Could you check a few things on this model? Use its own coordinates, in mm. Face numbers are marked on the shaded views. A direction names the side the tool comes from. Give positions to 0.01 mm unless a question says otherwise; leave off trailing zeros. Order: outer loops, then holes, each group sorted by start corner. A loop starts at its lowest first (then second) coordinate and runs counter-clockwise, first axis right, second up.
from build123d import *

# Parameters (mm, degrees)
F0_R     = 25
F1_DEPTH = 88
F3_DEPTH = 50
F5_DEPTH = 16
F7_R     = 6
F8_DEPTH = 9


with BuildPart() as f1:
    # F0 (on Top) → F1 (new body)
    with BuildSketch(Plane.XY):
        with BuildLine():
            Line((0, 75), (0, 0))
            Line((0, 0), (50, 0))
            ThreePointArc((50, 0), (87.5, 37.5), (50, 75))
            Line((50, 75), (0, 75))
        make_face()
        with Locations((50, 37.5)):
            Circle(F0_R, mode=Mode.SUBTRACT)
    extrude(amount=F1_DEPTH)

    # F2 (on Right) → F3 (join)
    with BuildSketch(Plane.YZ):
        Polygon((-25, 0), (0, 0), (0, 40), (-88, 40), (-88, 0), align=None)
        with BuildLine():
            ThreePointArc((-25, 31), (-14, 20), (-25, 9))
            Line((-25, 9), (-63, 9))
            ThreePointArc((-63, 9), (-74, 20), (-63, 31))
            Line((-63, 31), (-25, 31))
        make_face(mode=Mode.SUBTRACT)
    extrude(amount=F3_DEPTH)

    # F4 (on Right) → F5 (join)
    with BuildSketch(Plane.YZ):
        Polygon((-88, 40), (0, 40), (0, 88), align=None)
    extrude(amount=F5_DEPTH)

    # F7 (on face) → F8 (cut, through all)
    with BuildSketch(Plane.XY.offset(40)):
        with Locations((33, -44)):
            Circle(F7_R)
    extrude(amount=-F8_DEPTH, mode=Mode.SUBTRACT)


solid = f1.part
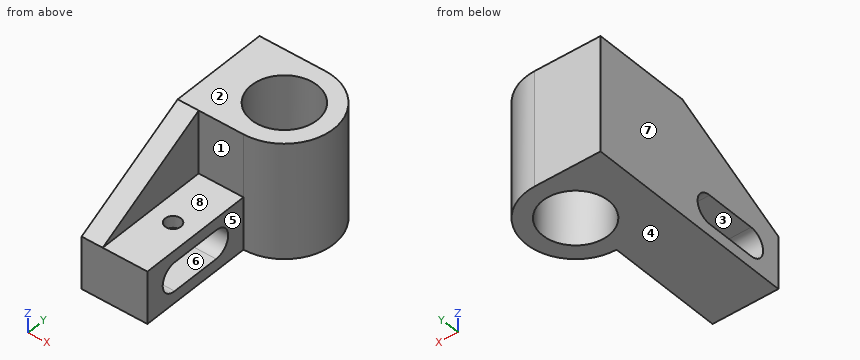
Item 1: We'd pull the mould along Y, two halves only. Please class the marked faces 1, 2 and 3: +Y half, -Y half, draft (parallel to the pull), parting line (faces both ways), or undercut.
Findings:
face 1: -Y half
face 2: draft
face 3: undercut
Item 2: Imagine slicing it at D-D on z = 62.5. List the corners of the cut face in (x, y) for me, then the cut area to 3 significant figures.
Findings:
outline: (0, -46.75) - (16, -46.75) - (16, 0) - (50, 0) arc R37.5 ccw to (50, 75) - (0, 75) - close; hole circle Ø50 at (50, 37.5)
area: 4,740 mm2
Item 3: For pin 1 (1.5 mm diameter, centred on x = 55.5, z = 48.5, fed in from -Y); pin 2 (3 mm diameter, centred on y = 45.5, z = 33, fed in from +X); pin 3 (19 mm diameter, centred on x = 33, y = -44, fed in from +Z), each with a flat end and sliding along its axis, tell me the tip position at first contact or that it passes through.
Findings:
pin 1: stops at y = 0.3
pin 2: stops at x = 86.93
pin 3: stops at z = 40
Item 4: Imagine slicing it at C-C on x = 6. List the corners of the cut face in (y, z) for me, then the cut area to 3 significant figures.
Findings:
outline: (-88, 0) - (75, 0) - (75, 88) - (0, 88) - (-88, 40) - close; hole (-63, 9) - (-25, 9) arc R11 ccw to (-25, 31) - (-63, 31) arc R11 ccw to start
area: 11,000 mm2
Item 5: Imagine slicing it at B-B on z = 20. List the corners of the cut face in (x, y) for me, then the cut area to 3 significant figures.
Findings:
outline: (0, -88) - (50, -88) - (50, -74) - (0, -74) - close; (0, -14) - (50, -14) - (50, 0) arc R37.5 ccw to (50, 75) - (0, 75) - close; hole circle Ø50 at (50, 37.5)
area: 5,400 mm2
Item 6: Please list where these lines run through material, in increasing order: line 1 along Y through (x, z) = (39.5, 20.5); line 2 along Y through (x, z) = (50, 41.5); line 3 along Y through (x, z) = (33, 34).
Findings:
line 1: y = -88 to -73.99, -14.01 to 14.81, 60.19 to 75
line 2: y = 0 to 12.5, 62.5 to 75
line 3: y = -88 to -50, -38 to 19.17, 55.83 to 75
Item 7: For the marked faces 4, 5, 6, 7 and 8, which set-ups out of +Z, -Z, +X, -X, +Y, -Y let a thin tool reach every point of the face, with its end or its side?
Findings:
face 4: -Z, +X, -X, +Y, -Y
face 5: +Z, -Z, +X, -Y
face 6: +X, -X
face 7: +Z, -Z, -X, +Y, -Y
face 8: +Z, +X, -Y
Item 8: Imagine slicing it at A-A on y = -44. List the corners of the cut face in (x, z) for me.
Findings:
outline: (0, 0) - (50, 0) - (50, 9) - (0, 9) - close; (0, 31) - (27, 31) - (27, 40) - (16, 40) - (16, 64) - (0, 64) - close; (39, 31) - (50, 31) - (50, 40) - (39, 40) - close
